Source: CAD feature listing. Evaluate the final solid. Frame: model axes, mm. A direction names the side the tool comes from. Give positions to 0.01 mm unless a question says otherwise; leave off trailing zeros. Order: outer loops, then holes, each group sorted by start corner. A loop starts at its lowest first (then second) coordinate and runs counter-clockwise, first axis right, second up. Notation, with made-up numbers: (60.25, 21.25) - (108.25, 21.25) arc R8 cw to (108.25, 34.25) - close; hole circle Ø6 at (14, 18). An arc over 180 degrees is marked (long way). One line per item, written item: value. Start each with the question number.
from build123d import *

# Parameters (mm, degrees)
EXTRUDE007_START                     = 4.5
SKETCH007_W                          = 4
SKETCH007_H                          = 3
EXTRUDE007_DEPTH                     = 0.5
EXTRUDE006_START                     = -4
SKETCH006_AS_DRAWN_W                 = 6
SKETCH006_AS_DRAWN_H                 = 1.5
EXTRUDE006_DEPTH                     = 4
EXTRUDE006_ONTO_SKETCH006_ROLL_ANGLE = 90
EXTRUDE005_DEPTH                     = 2
EXTRUDE003_START                     = -15
SKETCH003_AS_DRAWN_W                 = 7
SKETCH003_AS_DRAWN_H                 = 1.5
EXTRUDE003_DEPTH                     = 10
EXTRUDE003_ONTO_SKETCH003_ROLL_ANGLE = 90
EXTRUDE002_DEPTH                     = 6
EXTRUDE002_DEPTH_BACK                = 2
SKETCH_W                             = 26.5
SKETCH_H                             = 16
EXTRUDE001_DEPTH                     = 6
EXTRUDE001_DEPTH_BACK                = 0.5
EXTRUDE_DEPTH                        = 5
EXTRUDE_DEPTH_BACK                   = 1.5
FILLET_R                             = 1
CHAMFER_SIZE                         = 0.3


with BuildPart() as extrude007:
    # Sketch007 (on Cut) → Extrude007 (new body)
    with BuildSketch(Plane.XY.offset(EXTRUDE007_START)):
        with Locations((14.75, 5.419451)):
            Rectangle(SKETCH007_W, SKETCH007_H)
    extrude(amount=EXTRUDE007_DEPTH)


with BuildPart() as extrude006:
    # Sketch006 as drawn → Extrude006 (new)
    with BuildSketch(Plane.XY.offset(EXTRUDE006_START)):
        with Locations((14.75, 2.75)):
            Rectangle(SKETCH006_AS_DRAWN_W, SKETCH006_AS_DRAWN_H)
    extrude(amount=-EXTRUDE006_DEPTH)


with BuildPart() as extrude006_1:
    # Extrude006 onto Sketch006 roll: moved
    add(extrude006.part.rotate(Axis((0, 0, 0), (1, 0, 0)), EXTRUDE006_ONTO_SKETCH006_ROLL_ANGLE))


with BuildPart() as extrude006_2:
    # Extrude006 onto Sketch006 placement: moved
    add(extrude006_1.part)


with BuildPart() as extrude005:
    # Sketch005 → Extrude005 (new body)
    with BuildSketch(Plane.YZ):
        with BuildLine():
            Line((17, 5), (19.8, 5))
            Line((19.8, 5), (19.8, 1.7))
            ThreePointArc((18.6, 0.5), (19.448528, 0.851472), (19.8, 1.7))
            Line((18.6, 0.5), (18.2, 0.5))
            ThreePointArc((17, 1.7), (17.351472, 0.851472), (18.2, 0.5))
            Line((17, 1.7), (17, 5))
        make_face()
    extrude(amount=EXTRUDE005_DEPTH)


with BuildPart() as extrude003:
    # Sketch003 as drawn → Extrude003 (new)
    with BuildSketch(Plane.XY.offset(EXTRUDE003_START)):
        with Locations((8.25, 3.25)):
            Rectangle(SKETCH003_AS_DRAWN_W, SKETCH003_AS_DRAWN_H)
        with Locations((21.25, 3.25)):
            Rectangle(SKETCH003_AS_DRAWN_W, SKETCH003_AS_DRAWN_H)
    extrude(amount=-EXTRUDE003_DEPTH)


with BuildPart() as extrude003_1:
    # Extrude003 onto Sketch003 roll: moved
    add(extrude003.part.rotate(Axis((0, 0, 0), (1, 0, 0)), EXTRUDE003_ONTO_SKETCH003_ROLL_ANGLE))


with BuildPart() as extrude003_2:
    # Extrude003 onto Sketch003 placement: moved
    add(extrude003_1.part)


with BuildPart() as extrude002:
    # Sketch002 → Extrude002 (new body, two sides)
    with BuildSketch(Plane.XY) as extrude002_sk:
        with BuildLine():
            ThreePointArc((3.75, 26.5), (2.25, 25), (3.75, 23.5))
            Line((3.75, 23.5), (25.75, 23.5))
            ThreePointArc((25.75, 23.5), (27.25, 25), (25.75, 26.5))
            Line((3.75, 26.5), (25.75, 26.5))
        make_face()
        with BuildLine():
            ThreePointArc((3.628907, 4.5), (2.128907, 3), (3.628907, 1.5))
            Line((3.628907, 1.5), (25.628907, 1.5))
            ThreePointArc((25.628907, 1.5), (27.128907, 3), (25.628907, 4.5))
            Line((3.628907, 4.5), (25.628907, 4.5))
        make_face()
    extrude(amount=EXTRUDE002_DEPTH)
    extrude(extrude002_sk.sketch, amount=-EXTRUDE002_DEPTH_BACK)


with BuildPart() as extrude001:
    # Sketch → Extrude001 (new body, two sides)
    with BuildSketch(Plane.XY) as extrude001_sk:
        with Locations((14.75, 14.020797)):
            Rectangle(SKETCH_W, SKETCH_H)
    extrude(amount=EXTRUDE001_DEPTH)
    extrude(extrude001_sk.sketch, amount=-EXTRUDE001_DEPTH_BACK)


with BuildPart() as chamfer_body:
    # Sketch001 (on Sketch) → Extrude (new body, two sides)
    with BuildSketch(Plane.XY) as extrude_sk:
        with BuildLine():
            Line((3, 28), (26.5, 28))
            ThreePointArc((29.5, 25), (28.62132, 27.12132), (26.5, 28))
            Line((29.5, 25), (29.5, 3))
            ThreePointArc((26.5, 0), (28.62132, 0.87868), (29.5, 3))
            Line((26.5, 0), (3, 0))
            ThreePointArc((0, 3), (0.87868, 0.87868), (3, 0))
            Line((0, 3), (0, 25))
            ThreePointArc((3, 28), (0.87868, 27.12132), (0, 25))
        make_face()
    extrude(amount=EXTRUDE_DEPTH)
    extrude(extrude_sk.sketch, amount=-EXTRUDE_DEPTH_BACK)

    # Cut: cut Extrude001
    add(extrude001.part, mode=Mode.SUBTRACT)

    # Cut001: cut Extrude002
    add(extrude002.part, mode=Mode.SUBTRACT)

    # Cut002: cut Extrude003
    add(extrude003_2.part, mode=Mode.SUBTRACT)

    # Fillet
    fillet_edges = [chamfer_body.edges().sort_by_distance(p)[0] for p in [
        (0, 14, -1.5),
        (0, 14, 5),
        (0.87868, 0.87868, -1.5),
        (0.87868, 0.87868, 5),
        (0.87868, 27.12132, -1.5),
        (14.75, 0, -1.5),
        (14.75, 28, -1.5),
        (28.62132, 0.87868, -1.5),
        (28.62132, 27.12132, -1.5),
        (29.5, 14, -1.5),
        (14.75, 0, 5),
        (14.75, 28, 5),
        (28.62132, 0.87868, 5),
        (28.62132, 27.12132, 5),
        (29.5, 14, 5),
    ]]
    fillet(fillet_edges, radius=FILLET_R)

    # Cut004: cut Extrude005
    add(extrude005.part, mode=Mode.SUBTRACT)

    # Cut005: cut Extrude006
    add(extrude006_2.part, mode=Mode.SUBTRACT)

    # Cut006: cut Extrude007
    add(extrude007.part, mode=Mode.SUBTRACT)

    # Chamfer
    chamfer_edges = [chamfer_body.edges().sort_by_distance(p)[0] for p in [
        (12.75, 5.260399, 5),
        (16.75, 5.260399, 5),
    ]]
    chamfer(chamfer_edges, length=CHAMFER_SIZE)


solid = chamfer_body.part
1. Section C-C on z = 1. Return the cut outline in (x, y).
2. Section B-B on y = 11. Return the cut outline in (x, z).
3. Section A-A on x = 10. Return the cut outline in (y, z), then the cut area to 3 significant figures.
4. Draft query along Y for faces 5 (the flat face through (21, 23, 4)), 6 (the flat face through (14, 1.5, 2)), 7 (the cylindrical face through (14.914, 27.699, -1.215)), 8 (the flat face through (29.5, 14, 2)). Return one class per face: pulls with the +Y half, pulls with the -Y half, needs draft (parallel to the pull), parting line crosses it, or undercut.
5. Ray query, L1, parallel to Y at x = 7, z = 2; L2, parallel to Y at x = 23.75, z = 3.75; L3, parallel to Z at x = 7, y = 23. Return the intervals inside material, ascending.
6. Contact query for flat-ended pins moving along their axis: pin 1 Ø1.2 at (x, y) = (14, 5.5) entering from +Z; pin 2 Ø0.8 at (x, z) = (1, 4) entering from +Y; pin 3 Ø1.5 at (x, y) = (13, 8) entering from +Z. Output: stop coordinate, or through.
7. Set-up query: faces 1 (the flat face through (1, 19.8, 3)), 2 (the flat face through (15, 23.5, 1)), 3 (the flat face through (4.75, 23, 3)), 4 (the cylindrical face through (0.86, 0.9, 1.78)). Return all of +Z, -Z, +X, -X, +Y, -Y with unobstructed straight access to the full face (end or side cutting, diameter ignored); none if empty.
Data:
1. outline: (0, 3) arc R3 ccw to (3, 0) - (26.5, 0) arc R3 ccw to (29.5, 3) - (29.5, 25) arc R3 ccw to (26.5, 28) - (3, 28) arc R3 ccw to (0, 25) - (0, 19.57) - (1.5, 19.57) - (1.5, 22.02) - (28, 22.02) - (28, 6.02) - (1.5, 6.02) - (1.5, 17.23) - (0, 17.23) - close; hole (3.63, 1.5) - (25.63, 1.5) arc R1.5 ccw to (25.63, 4.5) - (3.63, 4.5) arc R1.5 ccw to start; hole (3.75, 23.5) - (25.75, 23.5) arc R1.5 ccw to (25.75, 26.5) - (3.75, 26.5) arc R1.5 ccw to start
2. outline: (0, -0.5) arc R1 ccw to (1, -1.5) - (28.5, -1.5) arc R1 ccw to (29.5, -0.5) - (29.5, 4) arc R1 ccw to (28.5, 5) - (28, 5) - (28, -0.5) - (1.5, -0.5) - (1.5, 5) - (1, 5) arc R1 ccw to (0, 4) - close
3. outline: (0, -0.5) arc R1 ccw to (1, -1.5) - (1.5, -1.5) - (1.5, 5) - (1, 5) arc R1 ccw to (0, 4) - close; (4.5, -1.5) - (23.5, -1.5) - (23.5, 2.5) - (22.02, 2.5) - (22.02, -0.5) - (6.02, -0.5) - (6.02, 5) - (4.5, 5) - close; (22.02, 4) - (23.5, 4) - (23.5, 5) - (22.02, 5) - close; (26.5, -1.5) - (27, -1.5) arc R1 ccw to (28, -0.5) - (28, 4) arc R1 ccw to (27, 5) - (26.5, 5) - close
3. area: 51.9 mm2
4. face 5: undercut
4. face 6: undercut
4. face 7: pulls with the +Y half
4. face 8: needs draft
5. L1: y = 0 to 1.5, 4.5 to 6.02, 22.02 to 23.5, 26.5 to 28
5. L2: y = 0 to 1.5, 4.5 to 6.02, 26.5 to 28
5. L3: z = -1.5 to 2.5, 4 to 5
6. pin 1: stops at z = 4.5
6. pin 2: stops at y = 27.54
6. pin 3: stops at z = -0.5
7. face 1: +Z, -X
7. face 2: +Z, -Z
7. face 3: none
7. face 4: +Z, -Z, -X, -Y
